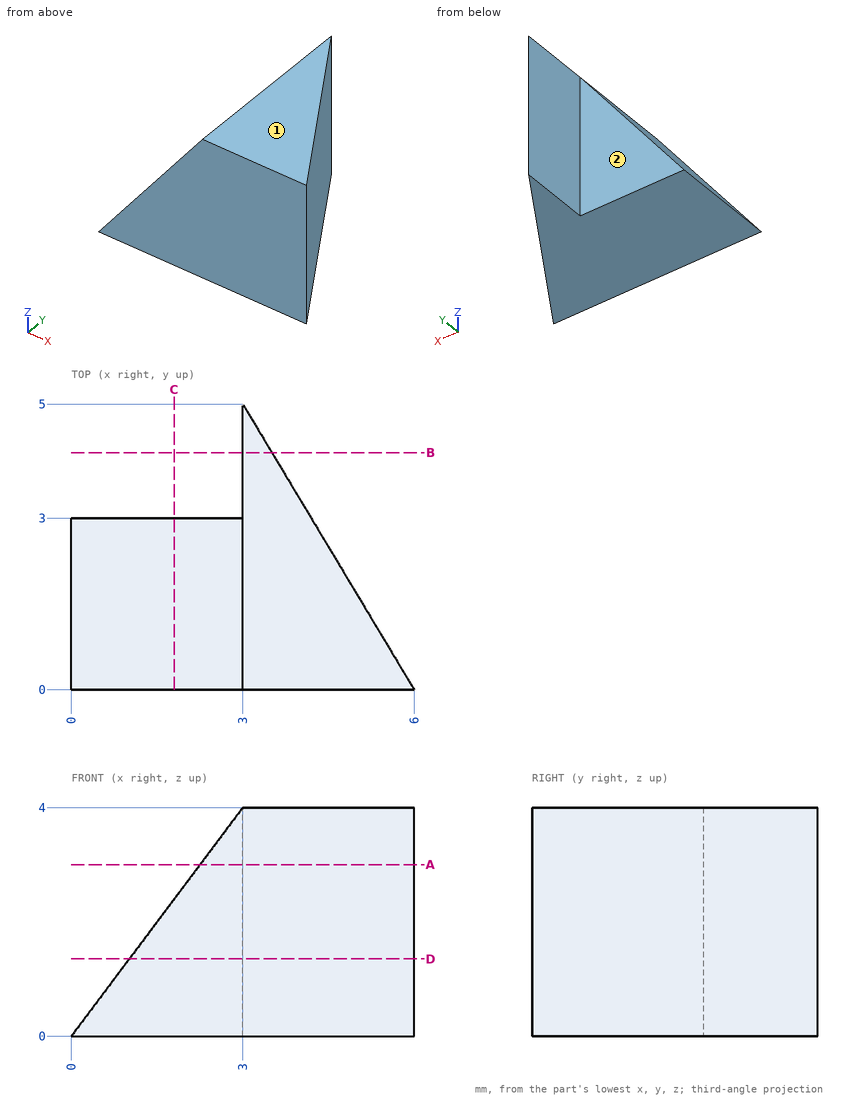
Geometry: see drawing. Coordinates: mm, zero at the bounding-box minimum. A direction names the side the tool comes from. Give positions to 0.01 mm unless a question says otherwise; leave off trailing zeros. Loops run counter-clockwise (first coordinate to the right, second up) from the corner with the lowest first, then second, coordinate; pieces in that order, holes last. Notation, with made-up numbers: (-19.75, 72) -> (22.25, 72) arc R12 ccw to (22.25, 88) -> close; hole circle Ø1 at (16, 70). An arc over 180 degrees is marked (long way). Use one line per item in the form item = value.
Item 1: Section query B-B on y = 4.15. Output: boundary loops of the cut face in (x, z), and give its area (3 significant figures).
A:
outline = (3, 0) -> (3.51, 0) -> (3.51, 4) -> (3, 4) -> close
area = 2.04 mm^2
Item 2: Line query: probe 1 along Y at (x, z) = (2.9, 1.7); probe 2 along Y at (x, z) = (3.8, 2.55); probe 3 along X at (y, z) = (0.35, 3.45). Output: solid intervals per line, ascending.
A:
probe_1 = 0 to 3
probe_2 = 0 to 3.67
probe_3 = 2.59 to 5.79
Item 3: Section query A-A on z = 3. Output: boundary loops of the cut face in (x, y), and give its area (3 significant figures).
A:
outline = (2.25, 0) -> (6, 0) -> (3, 5) -> (3, 3) -> (2.25, 3) -> close
area = 9.75 mm^2
Item 4: Section query D-D on z = 1.35. Output: boundary loops of the cut face in (x, y), and give its area (3 significant figures).
A:
outline = (1.01, 0) -> (6, 0) -> (3, 5) -> (3, 3) -> (1.01, 3) -> close
area = 13.5 mm^2
Item 5: Section query C-C on x = 1.8. Output: boundary loops of the cut face in (y, z), and give its area (3 significant figures).
A:
outline = (0, 0) -> (3, 0) -> (3, 2.4) -> (0, 2.4) -> close
area = 7.20 mm^2
Item 6: Pin query (flat end, axial travel): P1, Ø1, axis at x = 4.5, z = 1, coming from the -Y side; P2, Ø0.6, axis at y = 4.5, z = 2.5, coming from the -X side. Return the tip coordinate at first contact, or that it passes through.
A:
P1 = 0
P2 = 3
Item 7: Access query for the marked faces 1 and 2. Directions: +Z, -Z, +X, -X, +Y, -Y. A direction counts if a zero-diameter tool reaches every point of the face in a straight line with its end or side. Return the directions, or none.
A:
face_1 = +Z, +X, -X, +Y, -Y
face_2 = +Z, -Z, -X, +Y
